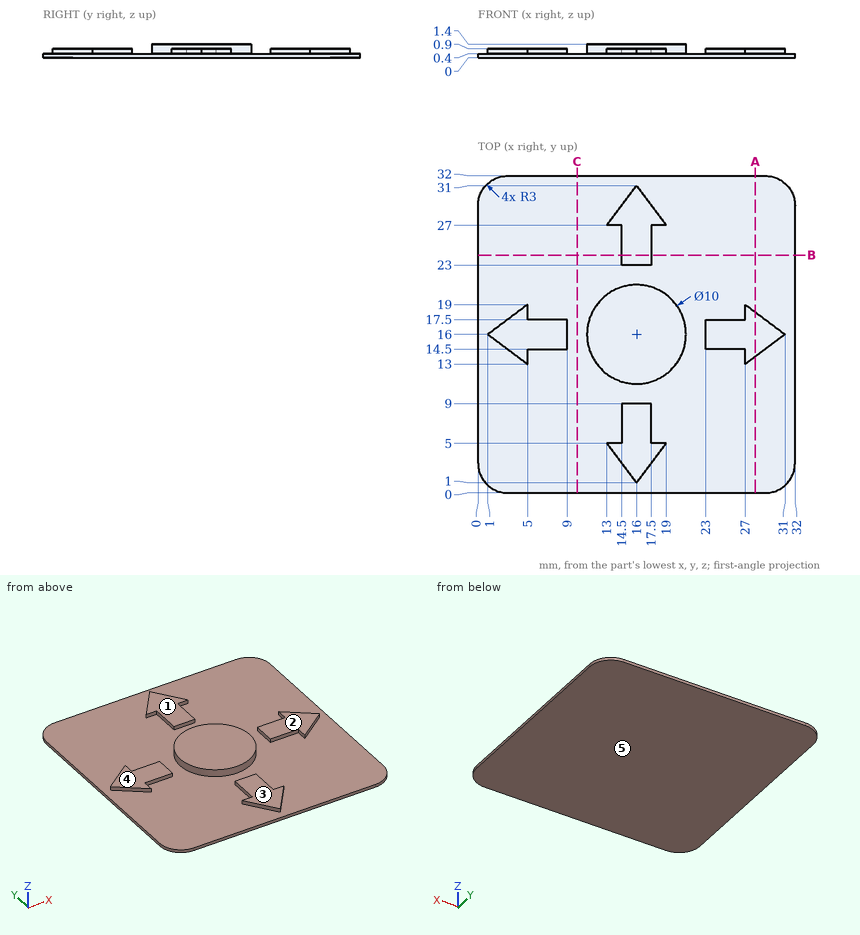
Input: dimensioned drawing with shaded views. Units: mm. Origin: part minimum x, y, z. A direction names the side the tool comes from. Round coordinates to 2 decimals unless told otherwise and drop trailing zeros. Order: outer loops, then holes, each group sorted by start corner. A loop starts at its lowest first (then second) coordinate and runs counter-clockwise, first axis right, second up.
Q1. Section C-C, the plane x = 10. Output: boundary loops of the cut face in (y, z).
Result sheet:
outline: (0, 0) - (32, 0) - (32, 0.4) - (0, 0.4) - close
Q2. Section A-A, the plane x = 28. Output: boundary loops of the cut face in (y, z).
Result sheet:
outline: (0, 0) - (32, 0) - (32, 0.4) - (18.25, 0.4) - (18.25, 0.9) - (13.75, 0.9) - (13.75, 0.4) - (0, 0.4) - close
Q3. Section B-B, the plane y = 24. Output: boundary loops of the cut face in (x, z), and give its area (3 significant figures).
Result sheet:
outline: (0, 0) - (32, 0) - (32, 0.4) - (17.5, 0.4) - (17.5, 0.9) - (14.5, 0.9) - (14.5, 0.4) - (0, 0.4) - close
area: 14.3 mm2
Q4. Material intervals for probe 1 along Y at (x, z) = (13.5, 0.5); probe 2 along Z at (x, y) = (2, 14); probe 3 along X at (y, z) = (8, 0.75), sorted ascending.
Result sheet:
probe 1: y = 4.33 to 5, 11.67 to 20.33, 27 to 27.67
probe 2: z = 0 to 0.4
probe 3: x = 14.5 to 17.5
Q5. Access query for the marked faces 1, 2, 3, 4 and 5. Directions: +Z, -Z, +X, -X, +Y, -Y. A direction counts if a zero-diameter tool reaches every point of the face in a straight line with its end or side. Return the directions, or none.
Result sheet:
face 1: +Z, +X, -X, +Y
face 2: +Z, +X, +Y, -Y
face 3: +Z, +X, -X, -Y
face 4: +Z, -X, +Y, -Y
face 5: -Z, +X, -X, +Y, -Y
Q6. Pin query (flat end, axial travel): pin 1 (6.5 mm diameter, centred on x = 5.5, y = 17.5, fed in from +Z). Return the tip coordinate at first contact, or that it passes through.
Result sheet:
pin 1: stops at z = 0.9
